```python
from build123d import *

# Parameters (mm, degrees)
SKETCH_1_R          = 12.75
SKETCH_1_R_2        = 3.15
EXTRUDE_1_DEPTH     = 1.6
SKETCH_3_W          = 2
SKETCH_3_H          = 5.467924172
CUT_EXTRUDE_3_DEPTH = 19.102071705


with BuildPart() as part:
    # Эскиз1 → Бобышка-Вытянуть1 (new body)
    with BuildSketch(Plane.XY):
        Circle(SKETCH_1_R)
        Circle(SKETCH_1_R_2, mode=Mode.SUBTRACT)
    extrude(amount=EXTRUDE_1_DEPTH)

    # Эскиз3 → Вырез-Вытянуть-Тонкостенный3 (cut, through all)
    with BuildSketch(Plane(origin=(0, 0, 0), x_dir=(-1, 0, 0), z_dir=(0, 0, -1))):
        with Locations((0, -10.016037914)):
            Rectangle(SKETCH_3_W, SKETCH_3_H)
        Polygon((-6.685244972, -10.902751931), (-3.471279784, -6.479108352), (-5.089313772, -5.303537847), (-8.303278961, -9.727181426), align=None)
        Polygon((-11.816953588, -4.891023195), (-6.616648674, -3.201341702), (-7.234682663, -1.299228669), (-12.434987577, -2.988910162), align=None)
        Polygon((-12.434987577, 2.988910162), (-7.234682663, 1.299228669), (-6.616648674, 3.201341702), (-11.816953588, 4.891023195), align=None)
        Polygon((-8.303278961, 9.727181426), (-5.089313772, 5.303537847), (-3.471279784, 6.479108352), (-6.685244972, 10.902751931), align=None)
        with Locations((0, 10.016037914)):
            Rectangle(SKETCH_3_W, SKETCH_3_H)
        Polygon((6.685244972, 10.902751931), (3.471279784, 6.479108352), (5.089313772, 5.303537847), (8.303278961, 9.727181426), align=None)
        Polygon((11.816953588, 4.891023195), (6.616648674, 3.201341702), (7.234682663, 1.299228669), (12.434987577, 2.988910162), align=None)
        Polygon((12.434987577, -2.988910162), (7.234682663, -1.299228669), (6.616648674, -3.201341702), (11.816953588, -4.891023195), align=None)
        Polygon((8.303278961, -9.727181426), (5.089313772, -5.303537847), (3.471279784, -6.479108352), (6.685244972, -10.902751931), align=None)
    extrude(amount=-CUT_EXTRUDE_3_DEPTH, mode=Mode.SUBTRACT)


solid = part.part
```
Design review of the part built by this model. Coordinates are the model's own, in mm. A direction names the side the tool comes from. Give positions to 0.01 mm unless a question says otherwise; leave off trailing zeros. Write each loop counter-clockwise with the first axis right and the second up, starting at its lowest first coordinate (ties: lowest second). Pieces come first, ordered by that corner, then holes. Notation, with made-up numbers: (28.5, 52.5) -> (57.5, 52.5) arc R18 ccw to (57.5, 71.5) -> close; hole circle Ø9 at (29, -17). An arc over 180 degrees is marked (long way). Answer in a Markdown table with one row per item.
(1) For faces 5 (the cylindrical face through (10.29, -7.53, 0.79)), 6 (the flat face through (-6.93, -2.24, 0.79)), 7 (the flat face through (9.23, -4.05, 0.79)), list the 3-axis set-ups (+Z, -Z, +X, -X, +Y, -Y) from which the entire face can be reached by the end or side of a thin tool; tool diameter is ignored.
Results:
| item | result |
|---|---|
| face 5 | +Z, -Z, +X, -Y |
| face 6 | +Z, -Z |
| face 7 | +Z, -Z, +X |
(2) Consider section A-A (x = 0). State the section outline as (y, z) points.
Results:
| item | result |
|---|---|
| outline | (-7.28, 0) -> (-3.15, 0) -> (-3.15, 1.6) -> (-7.28, 1.6) -> close; (3.15, 0) -> (7.28, 0) -> (7.28, 1.6) -> (3.15, 1.6) -> close |
(3) Consider section D-D (x = -9). State the section outline as (y, z) points, then the cut area to 3 significant figures.
Results:
| item | result |
|---|---|
| outline | (-9.03, 0) -> (-3.98, 0) -> (-3.98, 1.6) -> (-9.03, 1.6) -> close; (-1.87, 0) -> (1.87, 0) -> (1.87, 1.6) -> (-1.87, 1.6) -> close; (3.98, 0) -> (9.03, 0) -> (9.03, 1.6) -> (3.98, 1.6) -> close |
| area | 22.2 mm2 |
(4) Clearance check with flat-ended pins moving along their axes: pin 1 (0.8 mm diameter, centred on y = 9, z = 0.5, fed in from +X); pin 2 (0.8 mm diameter, centred on y = 11, z = 1, fed in from -X); pin 3 (0.5 mm diameter, centred on y = -10, z = 1, fed in from +X). State where each tip first meets the part, or that it passes through.
Results:
| item | result |
|---|---|
| pin 1 | x = 9.41 |
| pin 2 | x = -6.66 |
| pin 3 | x = 6.21 |
(5) Consider section C-C (y = 8). State the section outline as (x, z) points, then the cut area to 3 significant figures.
Results:
| item | result |
|---|---|
| outline | (-9.93, 0) -> (-7.05, 0) -> (-7.05, 1.6) -> (-9.93, 1.6) -> close; (-4.58, 0) -> (-1, 0) -> (-1, 1.6) -> (-4.58, 1.6) -> close; (1, 0) -> (4.58, 0) -> (4.58, 1.6) -> (1, 1.6) -> close; (7.05, 0) -> (9.93, 0) -> (9.93, 1.6) -> (7.05, 1.6) -> close |
| area | 20.7 mm2 |
(6) To check wall thickness, follow probe 1 along Y at (x, z) = (0, 0.55); probe 2 along X at (y, z) = (-9.5, 1.4); probe 3 along X at (y, z) = (-7.25, 0.2). State the ranges of each line that lie inside material, in increasing order.
Results:
| item | result |
|---|---|
| probe 1 | -7.28 to -3.15, 3.15 to 7.28 |
| probe 2 | -8.5 to -8.14, -5.67 to -1, 1 to 5.67, 8.14 to 8.5 |
| probe 3 | -10.49 to -6.5, -4.03 to 4.03, 6.5 to 10.49 |
(7) Consider section B-B (y = 0). State the section outline as (x, z) points, then the cut area to 3 significant figures.
Results:
| item | result |
|---|---|
| outline | (-12.75, 0) -> (-3.15, 0) -> (-3.15, 1.6) -> (-12.75, 1.6) -> close; (3.15, 0) -> (12.75, 0) -> (12.75, 1.6) -> (3.15, 1.6) -> close |
| area | 30.7 mm2 |
(8) Mouldability with a two-part tool opening along X and no side actions: class faces 1 (the cylindrical face through (-10.34, -7.46, 0.79)), 2 (the flat face through (9.162, 4.028, 0.789)), 3 (the flat face through (4.27, -5.9, 0.79)), 4 (the flat face through (-6.707, -7.53, 0.789)) as +X half, -X half, draft (parallel to the pull), parting line (faces both ways), or undercut.
Results:
| item | result |
|---|---|
| face 1 | -X half |
| face 2 | +X half |
| face 3 | undercut |
| face 4 | undercut |
